Input: part model. Units: mm. Frame: model coordinates. Face numbers are marked on the shaded views. A direction names the side the tool comes from. Round coordinates to 2 decimals unless told otherwise and drop trailing zeros. Loops run counter-clockwise (first coordinate to the right, second up) from the corner with the lowest first, then second, coordinate; pieces in that order, holes last. Notation, with made-up numbers: M 61.25,0 L 69.25,0 A15 ccw 69.25,21 Z; hole C 60,-24.5 d4. An arc over 180 degrees is marked long. Use one line per item in the form item = value. Start each with the question number.
Q1. Ray query, line 1 along X through (y, z) = (-7.5, 0); line 2 along X through (y, z) = (0.85, 0); line 3 along Z through (x, y) = (3.5, -3.75). Return the intervals inside material, ascending.
Q2. Mould query, pull axis Z, two halves, no side actions, for the marked faces 4, 5, 6 and 7. Classes: pulls with the +Z half, pulls with the -Z half, needs draft (parallel to the pull), parting line crosses it, or undercut.
Q3. Section query D-D, the plane x = -1. Output: boundary loops of the cut face in (y, z), and give its area (3 significant figures).
Q4. Access query for the marked faces 1, 2 and 3. Directions: +Z, -Z, +X, -X, +Y, -Y. A direction counts if a zero-diameter tool reaches every point of the face in a straight line with its end or side. Return the directions, or none.
Q5. Section query B-B, the plane x = 3.5. Output: boundary loops of the cut face in (y, z), and give its area (3 significant figures).
Q6. Section query A-A, the plane y = -4.25. Output: boundary loops of the cut face in (x, z), and give its area (3 significant figures).
Q7. First-contact query: P1, Ø5, axis at x = -2, y = -7.5, coming from the +Z side; P2, Ø4, axis at x = -9, y = -4.5, coming from the +Z side; P3, Ø12, axis at x = 7, y = -10, coming from the +Z side; P4, Ø13, axis at x = 0, z = 0, coming from the -Y side. Flat tips, straight axial feed; report the tip coordinate or a pass-through.
Q8. Section query C-C, the plane x = -8.75. Output: boundary loops of the cut face in (y, z), and give its area (3 significant figures).
```python
from build123d import *

# Parameters (mm, degrees)
SKETCH_3_R          = 10.188
CUT_EXTRUDE_1_DEPTH = 27.790856821
SKETCH_5_R          = 12.4
SKETCH_4_R          = 12.4
SKETCH_6_R          = 5
CUT_EXTRUDE_2_DEPTH = 30.478636501


with BuildPart() as part:
    # Эскиз2 → По сечениям1 section 0
    with BuildSketch(Plane(origin=(0, -18, 0), x_dir=(1, 0, 0), z_dir=(0, 1, 0))):
        with BuildLine():
            Line((-12.990381057, -7.5), (0, -15))
            Line((0, -15), (12.990381057, -7.5))
            Line((12.990381057, -7.5), (12.990381057, 7.5))
            Line((12.990381057, 7.5), (0, 15))
            Line((0, 15), (-12.990381057, 7.5))
            Line((-12.990381057, 7.5), (-12.990381057, -7.5))
        make_face()
    # Эскиз1 → По сечениям1 section 1
    with BuildSketch(Plane(origin=(0, 0, 0), x_dir=(1, 0, 0), z_dir=(0, 1, 0))):
        with BuildLine():
            Line((0, 15), (-12.990381057, 7.5))
            Line((-12.990381057, 7.5), (-12.990381057, -7.5))
            Line((-12.990381057, -7.5), (0, -15))
            Line((0, -15), (12.990381057, -7.5))
            Line((12.990381057, -7.5), (12.990381057, 7.5))
            Line((12.990381057, 7.5), (0, 15))
        make_face()
    loft()

    # Эскиз3 → Вырез-Вытянуть1 (cut, through all)
    with BuildSketch(Plane.XZ.offset(18)):
        with Locations(Location((0, 0, 0), (0, 0, 270))):
            Circle(SKETCH_3_R)
    extrude(amount=-CUT_EXTRUDE_1_DEPTH, mode=Mode.SUBTRACT)

    # Эскиз5 → По сечениям2 section 0
    with BuildSketch(Plane(origin=(0, 3.8, 0), x_dir=(1, 0, 0), z_dir=(0, 1, 0))):
        Circle(SKETCH_5_R)
    # Эскиз4 → По сечениям2 section 1
    with BuildSketch(Plane(origin=(0, 0, 0), x_dir=(1, 0, 0), z_dir=(0, 1, 0))):
        Circle(SKETCH_4_R)
    loft()

    # Эскиз6 → Вырез-Вытянуть2 (cut, through all)
    with BuildSketch(Plane(origin=(0, 3.8, 0), x_dir=(1, 0, 0), z_dir=(0, 1, 0))):
        with Locations(Location((0, 0, 0), (0, 0, 270))):
            Circle(SKETCH_6_R)
    extrude(amount=-CUT_EXTRUDE_2_DEPTH, mode=Mode.SUBTRACT)


solid = part.part
```
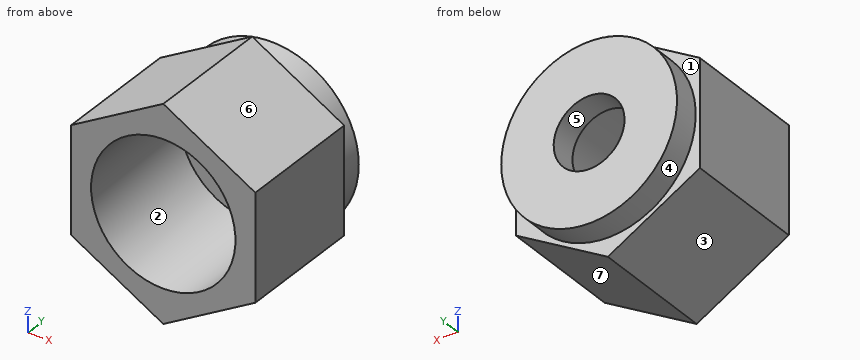
Results found:
q1.line_1 = -12.99 to -10.19, 10.19 to 12.99
q1.line_2 = -12.4 to -5, 5 to 12.4
q1.line_3 = -12.98 to -9.57, 9.57 to 12.98
q2.face_4 = parting line crosses it
q2.face_5 = undercut
q2.face_6 = pulls with the +Z half
q2.face_7 = pulls with the -Z half
q3.outline = M -18,-14.42 L 0,-14.42 L 0,-12.36 L 3.8,-12.36 L 3.8,-4.9 L 0,-4.9 L 0,-10.14 L -18,-10.14 Z; M -18,10.14 L 0,10.14 L 0,4.9 L 3.8,4.9 L 3.8,12.36 L 0,12.36 L 0,14.42 L -18,14.42 Z
q3.area = 211 mm²
q4.face_1 = +Y
q4.face_2 = -Y
q4.face_3 = -Z, -X, +Y, -Y
q5.outline = M -18,-12.98 L 0,-12.98 L 0,-11.9 L 3.8,-11.9 L 3.8,-3.57 L 0,-3.57 L 0,-9.57 L -18,-9.57 Z; M -18,9.57 L 0,9.57 L 0,3.57 L 3.8,3.57 L 3.8,11.9 L 0,11.9 L 0,12.98 L -18,12.98 Z
q5.area = 186 mm²
q6.outline = M -12.99,-7.5 L 0,-15 L 12.99,-7.5 L 12.99,7.5 L 0,15 L -12.99,7.5 Z; hole C 0,0 d20.38
q6.area = 258 mm²
q7.P1 = 15
q7.P2 = 10.96
q7.P3 = 14.42
q7.P4 = 0
q8.outline = M -18,-9.95 L 0,-9.95 L 0,-8.79 L 3.8,-8.79 L 3.8,8.79 L 0,8.79 L 0,9.95 L -18,9.95 L -18,5.22 L 0,5.22 L 0,-5.22 L -18,-5.22 Z
q8.area = 237 mm²
